```python
from build123d import *

# Parameters (mm, degrees)
F1_DEPTH    = 15
F2_W        = 46.8627084047
F2_H        = 56.3212386332
F3_DEPTH    = 13.30162
F4_W        = 13.7536320835
F4_H        = 12.7884671092
F5_DEPTH    = 13.81799
F6_T1_DEPTH = 75
F6_T3_DEPTH = 85.9022176913
F6_T5_DEPTH = 46.3573584799
F6_T7_DEPTH = 95


# Not quite as in the source:
# - a fillet or chamfer that OpenCascade refuses, or shapes differently, is made with other operations: its cross-section is extruded or revolved along the edge and cut away or added


with BuildPart() as f1:
    # F0 (on Top) → F1 (new body)
    with BuildSketch(Plane.XY):
        Polygon((-57.3696343694, 65.8665671945), (-57.3696343694, 4.9643495032), (-7.3696343694, 4.9643495032), (-7.3696343694, 74.9643495032), (-23.5122758895, 74.9643495032), (-23.5122758895, 65.8665671945), align=None)
    extrude(amount=F1_DEPTH)

    # F2 (on Top) → F3 (cut)
    with BuildSketch(Plane.XY):
        with Locations((-32.3047889397, 34.9865604658)):
            Rectangle(F2_W, F2_H)
    extrude(amount=F3_DEPTH, mode=Mode.SUBTRACT)

    # F4 (on Top) → F5 (cut)
    with BuildSketch(Plane.XY):
        with Locations((-15.8223016188, 69.8727704585)):
            Rectangle(F4_W, F4_H)
    extrude(amount=F5_DEPTH, mode=Mode.SUBTRACT)

    # F6: fillet of radius 5 on 6 edges, made by hand

    # F6_s2 → F6_t1 (cut)
    with BuildSketch(Plane.YZ.offset(-69.8696343694)):
        with BuildLine():
            ThreePointArc((4.9643495032, 10), (6.4288155972, 13.5355339059), (9.9643495032, 15))
            Line((9.9643495032, 15), (4.9643495032, 15))
            Line((4.9643495032, 15), (4.9643495032, 10))
        make_face()
        with BuildLine():
            ThreePointArc((4.9643495032, 5), (6.4288155972, 1.4644660941), (9.9643495032, 0))
            Line((9.9643495032, 0), (4.9643495032, 0))
            Line((4.9643495032, 0), (4.9643495032, 5))
        make_face()
    extrude(amount=F6_T1_DEPTH, mode=Mode.SUBTRACT)

    # F6_s4 → F6_t3 (cut)
    with BuildSketch(Plane.XZ.offset(-78.3665671945)):
        with BuildLine():
            ThreePointArc((-57.3696343694, 10), (-55.9051682753, 13.5355339059), (-52.3696343694, 15))
            Line((-52.3696343694, 15), (-57.3696343694, 15))
            Line((-57.3696343694, 15), (-57.3696343694, 10))
        make_face()
        with BuildLine():
            ThreePointArc((-57.3696343694, 5), (-55.9051682753, 1.4644660941), (-52.3696343694, 0))
            Line((-52.3696343694, 0), (-57.3696343694, 0))
            Line((-57.3696343694, 0), (-57.3696343694, 5))
        make_face()
    extrude(amount=F6_T3_DEPTH, mode=Mode.SUBTRACT)

    # F6_s6 → F6_t5 (cut)
    with BuildSketch(Plane.YZ.offset(-69.8696343694)):
        with BuildLine():
            ThreePointArc((65.8665671945, 10), (64.4021011004, 13.5355339059), (60.8665671945, 15))
            Line((60.8665671945, 15), (65.8665671945, 15))
            Line((65.8665671945, 15), (65.8665671945, 10))
        make_face()
    extrude(amount=F6_T5_DEPTH, mode=Mode.SUBTRACT)

    # F6_s8 → F6_t7 (cut)
    with BuildSketch(Plane.XZ.offset(-87.4643495032)):
        with BuildLine():
            ThreePointArc((-12.3696343694, 0), (-8.8341004635, 1.4644660941), (-7.3696343694, 5))
            Line((-7.3696343694, 5), (-7.3696343694, 0))
            Line((-7.3696343694, 0), (-12.3696343694, 0))
        make_face()
    extrude(amount=F6_T7_DEPTH, mode=Mode.SUBTRACT)


solid = f1.part
```
Geometry check sheet. Reference: the model listing, model coordinates, mm. A direction names the side the tool comes from. Give positions to 0.01 mm unless a question says otherwise; leave off trailing zeros. Loops run counter-clockwise (first coordinate to the right, second up) from the corner with the lowest first, then second, coordinate; pieces in that order, holes last. Notation, with made-up numbers: M 35.25,-4.5 L 75.25,-4.5 A17 ccw 75.25,11.5 Z; hole C -27,10.25 d10. An arc over 180 degrees is marked long. Answer as CSV lines item,"result".
Item 1: Cross-section at A-A on z = 6.5. Record the cut outline in (x, y), and give its area (3 significant figures).
Values:
outline,"M -57.37,4.96 L -7.37,4.96 L -7.37,74.96 L -8.95,74.96 L -8.95,63.48 L -22.7,63.48 L -22.7,74.96 L -23.51,74.96 L -23.51,65.87 L -57.37,65.87 Z; hole M -55.74,6.83 L -8.87,6.83 L -8.87,63.15 L -55.74,63.15 Z"
area,"395 mm²"
Item 2: Release check for a two-part mould opening along X. For faces 1 (the flat face through (-16, 69, 13.818)), 2 (the flat face through (-37, 64, 0)), 3 (the cylindrical face through (-56.924, 35.842, 2.937)), 4 (the flat face through (-7.37, 39, 10)) record: pulls with the +X half, pulls with the -X half, needs draft (parallel to the pull), parting line crosses it, or undercut.
Values:
face 1,"undercut"
face 2,"needs draft"
face 3,"pulls with the -X half"
face 4,"pulls with the +X half"
Item 3: Depth check by flat-ended pin: P1, Ø2, axis at x = -14.5, z = 6, coming from the +Y side; P2, Ø8, axis at x = -32, z = 3.5, coming from the +Y side; P3, Ø3, axis at y = 49.5, z = 2, coming from the -X side. Enter the tip coordinate at first touch or a pass-through.
Values:
P1,"stops at y = 63.48"
P2,"stops at y = 65.87"
P3,"stops at x = -57.14"
Item 4: Access from +Z, -Z, +X, -X, +Y, -Y to the whole of each face (thin tool, end or side, straight path). Record for faces 5 (the cylindrical face through (-40.68, 64.44, 13.5)), 6 (the flat face through (-8.873, 35, 7)), 7 (the flat face through (-14, 74.964, 14)), 8 (the flat face through (-16, 63.479, 7)), 9 (the flat face through (-40, 65.867, 5)).
Values:
face 5,"+Z, -X, +Y"
face 6,"-Z"
face 7,"+Z, -Z, +X, -X, +Y"
face 8,"-Z, +Y"
face 9,"+Z, -Z, -X, +Y"
Item 5: Cross-section at C-C on x = -25. Record the cut outline in (y, z), and give its area (3 significant figures).
Values:
outline,"M 4.96,5 A5 ccw 6.83,1.11 L 6.83,13.3 L 63.15,13.3 L 63.15,0 L 65.87,0 L 65.87,10 A5 ccw 60.87,15 L 9.96,15 A5 ccw 4.96,10 Z"
area,"149 mm²"
Item 6: Material ranges on line 1 (X direction, y = 68, z = 13.75); line 2 (X direction, y = 55.5, z = 9.5); line 3 (Y direction, x = -9.5, z = 6.75), recorded low to high.
Values:
line 1,"x = -23.51 to -22.7, -8.95 to -7.37"
line 2,"x = -57.37 to -55.74, -8.87 to -7.37"
line 3,"y = 4.96 to 6.83, 63.15 to 63.48"
Item 7: Cross-section at D-D on y = 48. Record the cut outline in (x, z), and give its area (3 significant figures).
Values:
outline,"M -57.37,5 A5 ccw -55.74,1.3 L -55.74,13.3 L -8.87,13.3 L -8.87,1.43 A5 ccw -7.37,5 L -7.37,15 L -52.37,15 A5 ccw -57.37,10 Z"
area,"113 mm²"
Item 8: Cross-section at B-B on y = 68. Record the cut outline in (x, z), and give its area (3 significant figures).
Values:
outline,"M -23.51,0 L -22.7,0 L -22.7,13.82 L -8.95,13.82 L -8.95,1.36 A5 ccw -7.37,5 L -7.37,15 L -23.51,15 Z"
area,"48.2 mm²"
